Autodesk Inventor part; units mm, degrees
ref_plane "YZ Plane" through (0, 0, 0) normal (1, 0, 0) x (0, 1, 0)
ref_plane "XZ Plane" through (0, 0, 0) normal (0, 1, 0) x (-1, 0, 0)
ref_plane "XY Plane" through (0, 0, 0) normal (0, 0, 1) x (1, 0, 0)
sketch "Sketch1" plane through (0, 0, 0) normal (0, 0, 1) x (1, 0, 0)
  line L0 (0, 0) -> (35.75, 0)
  line L1 (35.75, 0) -> (35.75, 12)
  line L2 (35.75, 12) -> (0, 12)
  line L3 (0, 12) -> (0, 0)
  dimension "d0" = 35.75
  dimension "d1" = 12
extrude "Extrusion1" add sketch "Sketch1" along normal blind 11
sketch "Sketch5" plane through (0, 0, 0) normal (0, 0, -1) x (-1, 0, 0)
  line L0 (0, 12) -> (0, 0)
  line L1 (-35.75, 0) -> (-35.75, 12)
  line L2 (0, 0) -> (-35.75, 0)
  line L3 (-35.75, 12) -> (0, 12)
  line L4 (-35.75, 6) -> (0, 6) construction
  line L5 (-30.75, 12) -> (-30.75, 0) construction
  line L6 (-23.75, 12) -> (-23.75, 0) construction
  line L7 (-16.75, 12) -> (-16.75, 0) construction
  point P0 (-30.75, 6)
  point P1 (-23.75, 6)
  point P2 (-16.75, 6)
  dimension "d46" = 6
  dimension "d48" = 5
  dimension "d49" = 7
  dimension "d50" = 7
hole "Hole3" at (30.75, 6, 0) at (23.75, 6, 0) at (16.75, 6, 0) direction (0, 0, 1) diameter 2.459 depth 8 tip angle 118
sketch "Sketch6" plane through (0, 0, 0) normal (0, 0, -1) x (-1, 0, 0)
  line L0 (0, 12) -> (0, 0)
  line L1 (-35.75, 0) -> (-35.75, 12)
  line L2 (0, 6) -> (-35.75, 6) construction
  point P0 (-6, 6)
  dimension "d35" = 6
hole "Hole4" at (6, 6, 0) direction (0, 0, 1) diameter 8 end through all
sketch "Sketch7" plane through (0, 0, 0) normal (0, 0, -1) x (-1, 0, 0)
  circle A0 centre (-6, 6) radius 4
  line L0 (0, 0) -> (-35.75, 0)
  line L1 (0, 12) -> (-12, 12)
  line L2 (-12, 12) -> (-12, 0)
  line L3 (-12, 0) -> (0, 0)
  line L4 (0, 0) -> (0, 12)
  dimension "d43" = 12
extrude "Extrusion3" cut sketch "Sketch7" against normal blind 9
fillet "Fillet5" radius 6 2 edges at (0, 12, 10) (0, 0, 10)
properties part number "termination_lv_conductor" material "Copper, Cast"
CAD build for the part. Positions are in the model's coordinates, mm. A direction names the side the tool comes from. Round coordinates to 2 decimals unless told otherwise and drop trailing zeros. Order: outer loops, then holes, each group sorted by start corner. A loop starts at its lowest first (then second) coordinate and runs counter-clockwise, first axis right, second up. Notation, with made-up numbers: (66.5, -0.5) - (94.5, -0.5) arc R27 ccw to (94.5, 36.5) - close; hole circle Ø11 at (-38.5, 17.25). An arc over 180 degrees is marked (long way). Answer in a Markdown table with one row per item. Add a question column.
(1) Probe L1, parallel to X at y = 6, z = 2.75; L2, parallel to X at y = 6, z = 9.9; L3, parallel to Y at x = 16.75, z = 4.25. List the from-to ranges inside material, lowest first. Write a range as [from, to].
(2) Drop flat-ended pins along their axis: pin 1 Ø6 at (x, y) = (15.5, 3.5) entering from -Z; pin 2 Ø4.5 at (y, z) = (8, 3) entering from -X; pin 3 Ø6 at (y, z) = (9.5, 9.5) entering from -X. Give the stop position or say it passes through.
(3) 3-axis set-ups, long thin cutter, end or side, ignore diameter. For faces 1 (the face through (12, 6, 4)), 2 (the face through (1.804, 10.289, 10.014)), 3 (the face through (15.53, 5.84, 4.06)): which of +Z, -Z, +X, -X, +Y, -Y reach the whole face in a straight line?
(4) Mould opens along Y. For faces 4 (the face through (10.1, 4.8, 9)), 5 (the face through (23.54, 5.95, 8.61)), 6 (the face through (24, 12, 5)) say: +Y half, -Y half, draft (parallel to the pull), parting line (faces both ways), or undercut.
(5) Band-saw the part on B-B on y = 9.25. List the corners of the cut face in (x, z).
(6) Band-saw the part on C-C on y = 1. List the corners of the cut face in (x, z), and give its area (3 significant figures).
(7) Band-saw the part on A-A on z = 1.25. List the corners of the cut face in (x, y).
Data:
| question | item | result |
|---|---|---|
| 1 | L1 | x = [12, 15.52], [17.98, 22.52], [24.98, 29.52], [31.98, 35.75] |
| 1 | L2 | x = [0, 2], [10, 35.75] |
| 1 | L3 | y = [0, 4.77], [7.23, 12] |
| 2 | pin 1 | stops at z = 0 |
| 2 | pin 2 | stops at x = 12 |
| 2 | pin 3 | stops at x = 0.02 |
| 3 | face 1 | -Z, -X, +Y, -Y |
| 3 | face 2 | +Z, -Z, -X, +Y |
| 3 | face 3 | -Z |
| 4 | face 4 | draft |
| 4 | face 5 | undercut |
| 4 | face 6 | +Y half |
| 5 | outline | (0.96, 9) - (3.67, 9) - (3.67, 11) - (0.96, 11) - close; (8.33, 9) - (12, 9) - (12, 0) - (35.75, 0) - (35.75, 11) - (8.33, 11) - close |
| 6 | outline | (2.68, 9) - (12, 9) - (12, 0) - (35.75, 0) - (35.75, 11) - (2.68, 11) - close |
| 6 | area | 280 mm^2 |
| 7 | outline | (12, 0) - (35.75, 0) - (35.75, 12) - (12, 12) - close; hole circle Ø2.46 at (16.75, 6); hole circle Ø2.46 at (23.75, 6); hole circle Ø2.46 at (30.75, 6) |
